```python
from build123d import *

# Parameters (mm, degrees)
BASPROSKE_W         = 6.35
BASPROSKE_H         = 26.9875
TOOTHCUT_DEPTH      = 39.690732902
TEETHCUTS_COUNT     = 15
BORSKE_R            = 1.5875
BORE_DEPTH          = 50.8000508
SKETCH1_R           = 6.35
BOSS_EXTRUDE1_DEPTH = 12.7
CUT_EXTRUDE1_DEPTH  = 43.603765196


with BuildPart() as part:
    # BasProSke → Base-Revolve (revolve)
    with BuildSketch(Plane(origin=(0, 0, 0), x_dir=(1, 0, 0), z_dir=(0, 1, 0)), mode=Mode.PRIVATE) as base_revolve_sk:
        with Locations((3.175, 13.49375)):
            Rectangle(BASPROSKE_W, BASPROSKE_H)
    revolve(base_revolve_sk.sketch.rotate(Axis((-10, 0, 0), (1, 0, 0)), 180), axis=Axis((-10, 0, 0), (1, 0, 0)))

    # TooCutSke → ToothCut (cut, through all)
    with BuildSketch(Plane(origin=(0, 0, 0), x_dir=(0, 0, -1), z_dir=(1, 0, 0))):
        with BuildLine():
            ThreePointArc((1.678565227, 19.771353806), (0, 19.84248), (-1.678565227, 19.771353806))
            ThreePointArc((-1.678565227, 19.771353806), (-2.61022813, 23.500276553), (-4.939797818, 26.557393771))
            ThreePointArc((-4.939797818, 26.557393771), (0, 27.0129), (4.939797818, 26.557393771))
            ThreePointArc((4.939797818, 26.557393771), (2.61022813, 23.500276553), (1.678565227, 19.771353806))
        make_face()
    toothcut = extrude(amount=TOOTHCUT_DEPTH, mode=Mode.SUBTRACT)

    # TeethCuts: ToothCut ×15 about axis
    teethcuts_axis = Axis((0, 0, 0), (1, 0, 0))
    for i in range(1, TEETHCUTS_COUNT):
        add(toothcut.rotate(teethcuts_axis, i * 360 / TEETHCUTS_COUNT), mode=Mode.SUBTRACT)

    # BorSke → Bore (cut, symmetric)
    with BuildSketch(Plane(origin=(0, 0, 0), x_dir=(0, 0, -1), z_dir=(1, 0, 0))):
        with Locations(Location((0, 0, 0), (0, 0, 180))):
            Circle(BORSKE_R)
    extrude(amount=BORE_DEPTH, both=True, mode=Mode.SUBTRACT)

    # Sketch1 → Boss-Extrude1 (add)
    with BuildSketch(Plane(origin=(6.35, 0, 0), x_dir=(0, 0, -1), z_dir=(1, 0, 0))):
        with Locations(Location((0, 0, 0), (0, 0, 180))):
            Circle(SKETCH1_R)
    extrude(amount=BOSS_EXTRUDE1_DEPTH)

    # Sketch2 → Cut-Extrude1 (cut, through all)
    with BuildSketch(Plane(origin=(19.05, 0, 0), x_dir=(0, 0, -1), z_dir=(1, 0, 0))):
        with BuildLine():
            ThreePointArc((2.286, 1.373715036), (1.313238554, 2.321269803), (0, 2.667))
            Line((0, 2.667), (0, 0))
            Line((0, 0), (2.286, 0))
            Line((2.286, 0), (2.286, 1.373715036))
        make_face()
        with BuildLine():
            Line((2.286, 0), (0, 0))
            Line((0, 0), (0, -2.667))
            ThreePointArc((0, -2.667), (1.313238554, -2.321269803), (2.286, -1.373715036))
            Line((2.286, -1.373715036), (2.286, 0))
        make_face()
        with BuildLine():
            Line((0, 0), (0, 2.667))
            ThreePointArc((0, 2.667), (-2.667, 0), (0, -2.667))
            Line((0, -2.667), (0, 0))
        make_face()
        with BuildLine():
            ThreePointArc((2.286, 1.373715036), (1.313238554, 2.321269803), (0, 2.667))
            Line((0, 2.667), (0, 0))
            Line((0, 0), (2.286, 0))
            Line((2.286, 0), (2.286, 1.373715036))
        make_face()
        with BuildLine():
            Line((2.286, 0), (0, 0))
            Line((0, 0), (0, -2.667))
            ThreePointArc((0, -2.667), (1.313238554, -2.321269803), (2.286, -1.373715036))
            Line((2.286, -1.373715036), (2.286, 0))
        make_face()
    extrude(amount=-CUT_EXTRUDE1_DEPTH, mode=Mode.SUBTRACT)


solid = part.part
```
Geometry check sheet. Reference: the model listing, model coordinates, mm. A direction names the side the tool comes from. Give positions to 0.01 mm unless a question says otherwise; leave off trailing zeros. Order: outer loops, then holes, each group sorted by start corner. A loop starts at its lowest first (then second) coordinate and runs counter-clockwise, first axis right, second up. Notation, with made-up numbers: (44.5, 39.25) - (97.5, 39.25) arc R18 ccw to (97.5, 69.25) - close; hole circle Ø5 at (-13.5, 56.5). An arc over 180 degrees is marked (long way). Answer in a Markdown table with one row per item. Add a question column.
Q1. Cross-section at B-B, the plane x = 17.25. Enter the section's corners in (y, z), then the cut area to 3 significant figures.
Q2. Material ranges on probe 1 along X at (y, z) = (15, 13); probe 2 along Y at (x, z) = (1, 10.5); probe 3 along Z at (x, y) = (1, 24), recorded low to high. Write a range as from..to.
Q3. Gauge pin test, flat ends, axial feed: pin 1 (3 mm diameter, centred on y = 18, z = -8.5, fed in from +X); pin 2 (3 mm diameter, centred on x = 10.5, z = 4.5, fed in from +Y); pin 3 (3 mm diameter, centred on x = 12.5, y = 0, fed in from +Z). Record the tip position at first contact, or that the pin passes through.
Q4. Tool access check on faces 4 (the cylindrical face through (3.131, 23.534, -2.627)), 5 (the cylindrical face through (3.131, -9.492, 21.695)). Record the directions out of +Z, -Z, +X, -X, +Y, -Y that give a thin tool (end or side, any length) a straight path to the whole face; none if there is none.
Q5. Cross-section at C-C, the plane y = -7. Enter the section's corners in (x, z).
Q6. Mould release check, pull along Z, two halves, no side actions. Record for faces 1 (the cylindrical face through (3.1, 9.8, 21.6)), 2 (the cylindrical face through (3.219, -8.349, -25.664)), 3 (the cylindrical face through (3.13, 20.43, -11.97)): pulls with the +Z half, pulls with the -Z half, needs draft (parallel to the pull), parting line crosses it, or undercut.
Q7. Cross-section at A-A, the plane y = -22. Enter the section's corners in (x, z), then the cut area to 3 significant figures.
Check values:
| question | item | result |
|---|---|---|
| 1 | outline | circle Ø12.7 at (0, 0); hole (-1.37, -2.29) - (1.37, -2.29) arc R2.67 ccw (long way) to start |
| 1 | area | 105 mm^2 |
| 2 | probe 1 | x = 0..6.35 |
| 2 | probe 2 | y = -24.86..-17.36, -16.84..18.88 |
| 2 | probe 3 | z = -7.02..-2.87, 2.87..7.02 |
| 3 | pin 1 | stops at x = 6.35 |
| 3 | pin 2 | stops at y = 5.6 |
| 3 | pin 3 | stops at z = 6.35 |
| 4 | face 4 | +X, -X, +Y |
| 4 | face 5 | +X, -X |
| 5 | outline | (0, -25.36) - (6.35, -25.36) - (6.35, 25.36) - (0, 25.36) - close |
| 6 | face 1 | pulls with the +Z half |
| 6 | face 2 | pulls with the -Z half |
| 6 | face 3 | undercut |
| 7 | outline | (0, -11.85) - (6.35, -11.85) - (6.35, -7.12) - (0, -7.12) - close; (0, -2.58) - (6.35, -2.58) - (6.35, 2.58) - (0, 2.58) - close; (0, 7.12) - (6.35, 7.12) - (6.35, 11.85) - (0, 11.85) - close |
| 7 | area | 92.9 mm^2 |
